from build123d import *

# Parameters (mm, degrees)
CUT_EXTRUDE1_DEPTH = 0.25


with BuildPart() as part:
    # Sketch1 → Revolve1 (revolve)
    with BuildSketch(Plane(origin=(0, 0, 0), x_dir=(0, 0, -1), z_dir=(1, 0, 0))):
        Polygon((0, 1), (0, 2), (-1.6, 2), (-1.6, 0), (5, 0), (5, 1), align=None)
    revolve(axis=Axis((0, 0, -5), (0, 0, 1)))

    # Sketch2 → Cut-Extrude1 (cut)
    with BuildSketch(Plane.XY.offset(1.6)):
        Polygon((-2, -0.25), (-0.25, -0.25), (-0.25, -2), (0, -2.25), (0.25, -2), (0.25, -0.25), (2, -0.25), (2.364373172, -0.114373172), (2, 0.25), (0.25, 0.25), (0.25, 2), (0, 2.480239465), (-0.25, 2), (-0.25, 0.25), (-2, 0.25), (-2.25, 0), align=None)
    extrude(amount=-CUT_EXTRUDE1_DEPTH, mode=Mode.SUBTRACT)


solid = part.part
The listing builds one solid part. Answer for the finished solid, in the listing's coordinates (mm). A direction names the side the tool comes from. Round coordinates to 2 decimals unless told otherwise and drop trailing zeros. Write each loop counter-clockwise with the first axis right and the second up, starting at its lowest first coordinate (ties: lowest second). Pieces come first, ordered by that corner, then holes. Notation, with made-up numbers: M 25,43.5 L 48,43.5 A31 ccw 48,79.5 Z; hole C -20,-6 d9. An arc over 180 degrees is marked long. Write each question's results on one line, items separated by ' | '. Start each with the question number.
(1) Find the intervals of material crossed by line 1 (Z direction, x = -0.6, y = -1.5); line 2 (Z direction, x = 1.35, y = 0); line 3 (Y direction, x = -0.85, z = 0.75), in increasing order.
(2) The part is cut by section A-A, the plane y = 0. Write down the section's boundary in (x, z), and give its area (3 significant figures).
(3) The part is cut by section C-C, the plane z = 1. Write down the section's boundary in (x, y), and give its area (3 significant figures).
(4) For faces 1 (the flat face through (1, 1, 1.6)), 2 (the flat face through (1, -1, 0)), determine the directions among +Z, -Z, +X, -X, +Y, -Y from which every point of the face is accessible in a straight line to the end or side of a thin tool.
(5) This flat-tipped pin is pushed along its axis until it touches: P1, Ø1, axis at x = -0.5, z = -4, coming from the +Y side. Where does it stop, or does it pass through?
(6) The part is cut by section D-D, the plane y = -1.6. Write down the section's boundary in (x, z).
(7) Determine the mould class of faces 3 (the flat face through (0, 0, 1.35)), 4 (the cylindrical face through (1, 0, -2)), 5 (the flat face through (-1, -1, 1.6)) for opening direction X: +X half, -X half, draft (parallel to the pull), parting line (faces both ways), or undercut.
(8) The part is cut by section B-B, the plane x = 0.75. Write down the section's boundary in (y, z), and give its area (3 significant figures).
Worked answers:
1) line 1: z = 0 to 1.6 | line 2: z = 0 to 1.35 | line 3: y = -1.81 to 1.81
2) outline: M -2,0 L -1,0 L -1,-5 L 1,-5 L 1,0 L 2,0 L 2,1.35 L -2,1.35 Z | area: 15.4 mm²
3) outline: C 0,0 d4 | area: 12.6 mm²
4) face 1: +Z, +X, -X, +Y, -Y | face 2: -Z
5) P1: stops at y = 1
6) outline: M -1.2,0 L 1.2,0 L 1.2,1.6 L 0.25,1.6 L 0.25,1.35 L -0.25,1.35 L -0.25,1.6 L -1.2,1.6 Z
7) face 3: undercut | face 4: parting line | face 5: draft
8) outline: M -1.85,0 L -0.66,0 L -0.66,-5 L 0.66,-5 L 0.66,0 L 1.85,0 L 1.85,1.6 L 0.25,1.6 L 0.25,1.35 L -0.25,1.35 L -0.25,1.6 L -1.85,1.6 Z | area: 12.4 mm²
